from build123d import *

# Parameters (mm, degrees)
BOX001_W       = 2
BOX001_H       = 2
BOX001_DEPTH   = 10
BOX_W          = 16
BOX_H          = 3
BOX_DEPTH      = 5
CYLINDER_R     = 2
CYLINDER_DEPTH = 5


with BuildPart() as cube001:
    # Box001 → Box001 (new body)
    with BuildSketch(Plane(origin=(-1, -1, 0), x_dir=(1, 0, 0), z_dir=(0, 0, 1))):
        with Locations((1, 1)):
            Rectangle(BOX001_W, BOX001_H)
    extrude(amount=BOX001_DEPTH)


with BuildPart() as cube:
    # Box → Box (new body)
    with BuildSketch(Plane(origin=(-8, -1.5, 0), x_dir=(1, 0, 0), z_dir=(0, 0, 1))):
        with Locations((8, 1.5)):
            Rectangle(BOX_W, BOX_H)
    extrude(amount=BOX_DEPTH)


with BuildPart() as cut:
    # Cylinder → Cylinder (new body)
    with BuildSketch(Plane.XY):
        Circle(CYLINDER_R)
    extrude(amount=CYLINDER_DEPTH)

    # Fusion: union Cube
    add(cube.part)

    # Cut: cut Cube001
    add(cube001.part, mode=Mode.SUBTRACT)


solid = cut.part
Design review of the part built by this model. Coordinates are the model's own, in mm. A direction names the side the tool comes from. Round coordinates to 2 decimals unless told otherwise and drop trailing zeros. Write each loop counter-clockwise with the first axis right and the second up, starting at its lowest first coordinate (ties: lowest second). Pieces come first, ordered by that corner, then holes.
Item 1: Consider section B-B on z = 2.85. Give the boundary of the cut face in (x, y).
Item 2: Consider section C-C on x = 5.75. Give the boundary of the cut face in (y, z).
Item 3: Consider section A-A on y = -0.35. Give the boundary of the cut face in (x, z), and give its area (3 significant figures).
Item 4: Draft analysis for pull direction Y (two halves, no side actions). For faces 5 (the flat face through (1, 0, 2)), 6 (the flat face through (8, 0, 2)), 7 (the flat face through (-5, -1.5, 2)), state which applies: released by +Y, released by -Y, zero draft, split by the parting line, or undercut.
Item 5: For faces 1 (the flat face through (-5, 1.5, 2)), 2 (the flat face through (5, 1.5, 2)), 3 (the flat face through (5, -1.5, 2)), 4 (the flat face through (-1, 0, 2)), list the 3-axis set-ups (+Z, -Z, +X, -X, +Y, -Y) from which the entire face can be reached by the end or side of a thin tool; tool diameter is ignored.
Item 6: Consider section D-D on y = 1.75. Give the boundary of the cut face in (x, z), and give its area (3 significant figures).
Item 7: Wall thickness on L1, parallel to X at y = -0.3, z = 3.1; L2, parallel to Y at x = -5, z = 2.2; L3, parallel to Y at x = 0.25, z = 3.2: over which ranges is each line inside the solid? List them lowest first.
Item 8: For pin 1 Ø1.5 at (x, z) = (-4.5, 1.5) entering from +Y, flat-tipped, find the tip position at first contact; note if it passes through.
Check values:
1. outline: (-8, -1.5) - (-1.32, -1.5) arc R2 ccw to (1.32, -1.5) - (8, -1.5) - (8, 1.5) - (1.32, 1.5) arc R2 ccw to (-1.32, 1.5) - (-8, 1.5) - close; hole (-1, -1) - (1, -1) - (1, 1) - (-1, 1) - close
2. outline: (-1.5, 0) - (1.5, 0) - (1.5, 5) - (-1.5, 5) - close
3. outline: (-8, 0) - (-1, 0) - (-1, 5) - (-8, 5) - close; (1, 0) - (8, 0) - (8, 5) - (1, 5) - close
3. area: 70.0 mm2
4. face 5: undercut
4. face 6: zero draft
4. face 7: released by -Y
5. face 1: +Z, -Z, -X, +Y
5. face 2: +Z, -Z, +X, +Y
5. face 3: +Z, -Z, +X, -Y
5. face 4: +Z, -Z
6. outline: (-0.97, 0) - (0.97, 0) - (0.97, 5) - (-0.97, 5) - close
6. area: 9.68 mm2
7. L1: x = -8 to -1, 1 to 8
7. L2: y = -1.5 to 1.5
7. L3: y = -1.98 to -1, 1 to 1.98
8. pin 1: stops at y = 1.5
